```python
from build123d import *

# Parameters (mm, degrees)
BASE_FLANGE1_DEPTH = 2.3
CUT_EXTRUDE2_REACH = 26.82
SKETCH12_W         = 4.6
SKETCH12_H         = 2.3
SKETCH12_W_2       = 3.45
SKETCH6_W          = 3.3
SKETCH6_H          = 7
TAB1_DEPTH         = 2.3
CUT_EXTRUDE1_REACH = 30.373
SKETCH10_R         = 2.5
SKETCH10_R_2       = 1
TAB2_DEPTH         = 2.3


# Sheet-metal steps are written as plain solids
with BuildPart() as part:
    # Sketch1 → Base-Flange1 (new body)
    with BuildSketch(Plane(origin=(0, 0, 0), x_dir=(1, 0, 0), z_dir=(0, 1, 0))):
        with BuildLine():
            Line((-20.6, -10), (20.6, -10))
            ThreePointArc((20.6, -10), (22.014213562, -9.414213562), (22.6, -8))
            Line((22.6, -8), (22.6, 8))
            ThreePointArc((22.6, 8), (22.014213562, 9.414213562), (20.6, 10))
            Line((20.6, 10), (-20.6, 10))
            ThreePointArc((-20.6, 10), (-22.014213562, 9.414213562), (-22.6, 8))
            Line((-22.6, 8), (-22.6, -8))
            ThreePointArc((-22.6, -8), (-22.014213562, -9.414213562), (-20.6, -10))
        make_face()
    extrude(amount=-BASE_FLANGE1_DEPTH)

    # Sketch12 → Cut-Extrude2 (cut, up to next)
    with BuildSketch(Plane(origin=(0, 0, 0), x_dir=(1, 0, 0), z_dir=(0, 1, 0)), mode=Mode.PRIVATE) as cut_extrude2_sk1:
        with Locations((-13, 0)):
            Rectangle(SKETCH12_W, SKETCH12_H)
    cut_extrude2_tool1 = extrude(cut_extrude2_sk1.sketch, amount=-CUT_EXTRUDE2_REACH, mode=Mode.PRIVATE) & part.part
    # Sketch12 → Cut-Extrude2 (cut, up to next)
    with BuildSketch(Plane(origin=(0, 0, 0), x_dir=(1, 0, 0), z_dir=(0, 1, 0)), mode=Mode.PRIVATE) as cut_extrude2_sk2:
        with Locations((7.6, 0)):
            Rectangle(SKETCH12_W, SKETCH12_H)
    cut_extrude2_tool2 = extrude(cut_extrude2_sk2.sketch, amount=-CUT_EXTRUDE2_REACH, mode=Mode.PRIVATE) & part.part
    # Sketch12 → Cut-Extrude2 (cut, up to next)
    with BuildSketch(Plane(origin=(0, 0, 0), x_dir=(1, 0, 0), z_dir=(0, 1, 0)), mode=Mode.PRIVATE) as cut_extrude2_sk3:
        with Locations((-18.3, 3.8)):
            Rectangle(SKETCH12_W, SKETCH12_H)
    cut_extrude2_tool3 = extrude(cut_extrude2_sk3.sketch, amount=-CUT_EXTRUDE2_REACH, mode=Mode.PRIVATE) & part.part
    # Sketch12 → Cut-Extrude2 (cut, up to next)
    with BuildSketch(Plane(origin=(0, 0, 0), x_dir=(1, 0, 0), z_dir=(0, 1, 0)), mode=Mode.PRIVATE) as cut_extrude2_sk4:
        with Locations((18.3, 3.8)):
            Rectangle(SKETCH12_W, SKETCH12_H)
    cut_extrude2_tool4 = extrude(cut_extrude2_sk4.sketch, amount=-CUT_EXTRUDE2_REACH, mode=Mode.PRIVATE) & part.part
    # Sketch12 → Cut-Extrude2 (cut, up to next)
    with BuildSketch(Plane(origin=(0, 0, 0), x_dir=(1, 0, 0), z_dir=(0, 1, 0)), mode=Mode.PRIVATE) as cut_extrude2_sk5:
        with Locations((-18.3, -3.8)):
            Rectangle(SKETCH12_W, SKETCH12_H)
    cut_extrude2_tool5 = extrude(cut_extrude2_sk5.sketch, amount=-CUT_EXTRUDE2_REACH, mode=Mode.PRIVATE) & part.part
    # Sketch12 → Cut-Extrude2 (cut, up to next)
    with BuildSketch(Plane(origin=(0, 0, 0), x_dir=(1, 0, 0), z_dir=(0, 1, 0)), mode=Mode.PRIVATE) as cut_extrude2_sk6:
        with Locations((18.3, -3.8)):
            Rectangle(SKETCH12_W, SKETCH12_H)
    cut_extrude2_tool6 = extrude(cut_extrude2_sk6.sketch, amount=-CUT_EXTRUDE2_REACH, mode=Mode.PRIVATE) & part.part
    # Sketch12 → Cut-Extrude2 (cut, up to next)
    with BuildSketch(Plane(origin=(0, 0, 0), x_dir=(1, 0, 0), z_dir=(0, 1, 0)), mode=Mode.PRIVATE) as cut_extrude2_sk7:
        with Locations((-9.225, 7.6)):
            Rectangle(SKETCH12_W_2, SKETCH12_H)
    cut_extrude2_tool7 = extrude(cut_extrude2_sk7.sketch, amount=-CUT_EXTRUDE2_REACH, mode=Mode.PRIVATE) & part.part
    # Sketch12 → Cut-Extrude2 (cut, up to next)
    with BuildSketch(Plane(origin=(0, 0, 0), x_dir=(1, 0, 0), z_dir=(0, 1, 0)), mode=Mode.PRIVATE) as cut_extrude2_sk8:
        with Locations((-9.225, -7.6)):
            Rectangle(SKETCH12_W_2, SKETCH12_H)
    cut_extrude2_tool8 = extrude(cut_extrude2_sk8.sketch, amount=-CUT_EXTRUDE2_REACH, mode=Mode.PRIVATE) & part.part
    add(cut_extrude2_tool1.solids().sort_by_distance((-13, 0, 0))[0], mode=Mode.SUBTRACT)
    add(cut_extrude2_tool2.solids().sort_by_distance((7.6, 0, 0))[0], mode=Mode.SUBTRACT)
    add(cut_extrude2_tool3.solids().sort_by_distance((-18.3, 0, -3.8))[0], mode=Mode.SUBTRACT)
    add(cut_extrude2_tool4.solids().sort_by_distance((18.3, 0, -3.8))[0], mode=Mode.SUBTRACT)
    add(cut_extrude2_tool5.solids().sort_by_distance((-18.3, 0, 3.8))[0], mode=Mode.SUBTRACT)
    add(cut_extrude2_tool6.solids().sort_by_distance((18.3, 0, 3.8))[0], mode=Mode.SUBTRACT)
    add(cut_extrude2_tool7.solids().sort_by_distance((-9.225, 0, -7.6))[0], mode=Mode.SUBTRACT)
    add(cut_extrude2_tool8.solids().sort_by_distance((-9.225, 0, 7.6))[0], mode=Mode.SUBTRACT)

    # Sketch6 → Tab1 (add)
    with BuildSketch(Plane(origin=(0, 0, 0), x_dir=(1, 0, 0), z_dir=(0, 1, 0))):
        with Locations((-14.5, 13.5)):
            Rectangle(SKETCH6_W, SKETCH6_H)
        with Locations((14.5, 13.5)):
            Rectangle(SKETCH6_W, SKETCH6_H)
        with Locations((14.5, -13.5)):
            Rectangle(SKETCH6_W, SKETCH6_H)
        with Locations((-14.5, -13.5)):
            Rectangle(SKETCH6_W, SKETCH6_H)
    extrude(amount=-TAB1_DEPTH)

    # Sketch9 → Cut-Extrude1 (cut, up to next)
    with BuildSketch(Plane(origin=(0, 0, 0), x_dir=(1, 0, 0), z_dir=(0, 1, 0)), mode=Mode.PRIVATE) as cut_extrude1_sk1:
        Polygon((-12.85, 11.15), (-13.35, 11.15), (-13.35, 13.35), (-13.5, 13.35), (-13.5, 15.85), (-13.35, 15.85), (-13.35, 17), (-12.85, 17), align=None)
    cut_extrude1_tool1 = extrude(cut_extrude1_sk1.sketch, amount=-CUT_EXTRUDE1_REACH, mode=Mode.PRIVATE) & part.part
    # Sketch9 → Cut-Extrude1 (cut, up to next)
    with BuildSketch(Plane(origin=(0, 0, 0), x_dir=(1, 0, 0), z_dir=(0, 1, 0)), mode=Mode.PRIVATE) as cut_extrude1_sk2:
        Polygon((-16.15, 17), (-16.15, 11.15), (-15.65, 11.15), (-15.65, 13.35), (-15.5, 13.35), (-15.5, 15.85), (-15.65, 15.85), (-15.65, 17), align=None)
    cut_extrude1_tool2 = extrude(cut_extrude1_sk2.sketch, amount=-CUT_EXTRUDE1_REACH, mode=Mode.PRIVATE) & part.part
    # Sketch9 → Cut-Extrude1 (cut, up to next)
    with BuildSketch(Plane(origin=(0, 0, 0), x_dir=(1, 0, 0), z_dir=(0, 1, 0)), mode=Mode.PRIVATE) as cut_extrude1_sk3:
        Polygon((-16.15, -11.15), (-15.65, -11.15), (-15.65, -13.35), (-15.5, -13.35), (-15.5, -15.85), (-15.65, -15.85), (-15.65, -17), (-16.15, -17), align=None)
    cut_extrude1_tool3 = extrude(cut_extrude1_sk3.sketch, amount=-CUT_EXTRUDE1_REACH, mode=Mode.PRIVATE) & part.part
    # Sketch9 → Cut-Extrude1 (cut, up to next)
    with BuildSketch(Plane(origin=(0, 0, 0), x_dir=(1, 0, 0), z_dir=(0, 1, 0)), mode=Mode.PRIVATE) as cut_extrude1_sk4:
        Polygon((-12.85, -17), (-12.85, -11.15), (-13.35, -11.15), (-13.35, -13.35), (-13.5, -13.35), (-13.5, -15.85), (-13.35, -15.85), (-13.35, -17), align=None)
    cut_extrude1_tool4 = extrude(cut_extrude1_sk4.sketch, amount=-CUT_EXTRUDE1_REACH, mode=Mode.PRIVATE) & part.part
    # Sketch9 → Cut-Extrude1 (cut, up to next)
    with BuildSketch(Plane(origin=(0, 0, 0), x_dir=(1, 0, 0), z_dir=(0, 1, 0)), mode=Mode.PRIVATE) as cut_extrude1_sk5:
        Polygon((12.85, -11.15), (13.35, -11.15), (13.35, -13.35), (13.5, -13.35), (13.5, -15.85), (13.35, -15.85), (13.35, -17), (12.85, -17), align=None)
    cut_extrude1_tool5 = extrude(cut_extrude1_sk5.sketch, amount=-CUT_EXTRUDE1_REACH, mode=Mode.PRIVATE) & part.part
    # Sketch9 → Cut-Extrude1 (cut, up to next)
    with BuildSketch(Plane(origin=(0, 0, 0), x_dir=(1, 0, 0), z_dir=(0, 1, 0)), mode=Mode.PRIVATE) as cut_extrude1_sk6:
        Polygon((16.15, -17), (16.15, -11.15), (15.65, -11.15), (15.65, -13.35), (15.5, -13.35), (15.5, -15.85), (15.65, -15.85), (15.65, -17), align=None)
    cut_extrude1_tool6 = extrude(cut_extrude1_sk6.sketch, amount=-CUT_EXTRUDE1_REACH, mode=Mode.PRIVATE) & part.part
    # Sketch9 → Cut-Extrude1 (cut, up to next)
    with BuildSketch(Plane(origin=(0, 0, 0), x_dir=(1, 0, 0), z_dir=(0, 1, 0)), mode=Mode.PRIVATE) as cut_extrude1_sk7:
        Polygon((12.85, 17), (12.85, 11.15), (13.35, 11.15), (13.35, 13.35), (13.5, 13.35), (13.5, 15.85), (13.35, 15.85), (13.35, 17), align=None)
    cut_extrude1_tool7 = extrude(cut_extrude1_sk7.sketch, amount=-CUT_EXTRUDE1_REACH, mode=Mode.PRIVATE) & part.part
    # Sketch9 → Cut-Extrude1 (cut, up to next)
    with BuildSketch(Plane(origin=(0, 0, 0), x_dir=(1, 0, 0), z_dir=(0, 1, 0)), mode=Mode.PRIVATE) as cut_extrude1_sk8:
        Polygon((16.15, 11.15), (15.65, 11.15), (15.65, 13.35), (15.5, 13.35), (15.5, 15.85), (15.65, 15.85), (15.65, 17), (16.15, 17), align=None)
    cut_extrude1_tool8 = extrude(cut_extrude1_sk8.sketch, amount=-CUT_EXTRUDE1_REACH, mode=Mode.PRIVATE) & part.part
    add(cut_extrude1_tool1.solids().sort_by_distance((-13.136932, 0, -14.134659))[0], mode=Mode.SUBTRACT)
    add(cut_extrude1_tool2.solids().sort_by_distance((-15.863068, 0, -14.134659))[0], mode=Mode.SUBTRACT)
    add(cut_extrude1_tool3.solids().sort_by_distance((-15.863068, 0, 14.134659))[0], mode=Mode.SUBTRACT)
    add(cut_extrude1_tool4.solids().sort_by_distance((-13.136932, 0, 14.134659))[0], mode=Mode.SUBTRACT)
    add(cut_extrude1_tool5.solids().sort_by_distance((13.136932, 0, 14.134659))[0], mode=Mode.SUBTRACT)
    add(cut_extrude1_tool6.solids().sort_by_distance((15.863068, 0, 14.134659))[0], mode=Mode.SUBTRACT)
    add(cut_extrude1_tool7.solids().sort_by_distance((13.136932, 0, -14.134659))[0], mode=Mode.SUBTRACT)
    add(cut_extrude1_tool8.solids().sort_by_distance((15.863068, 0, -14.134659))[0], mode=Mode.SUBTRACT)

    # Sketch10 → Tab2 (add)
    with BuildSketch(Plane(origin=(0, 0, 0), x_dir=(1, 0, 0), z_dir=(0, 1, 0))):
        with Locations((-23.6, 0)):
            Circle(SKETCH10_R)
        with Locations(Location((-23.6, 0, 0), (0, 0, 270))):
            Circle(SKETCH10_R_2, mode=Mode.SUBTRACT)
    extrude(amount=-TAB2_DEPTH)


solid = part.part
```
Part model, mm, in its own coordinate system. A direction names the side the tool comes from. Give positions to 0.01 mm unless a question says otherwise; leave off trailing zeros. Order: outer loops, then holes, each group sorted by start corner. A loop starts at its lowest first (then second) coordinate and runs counter-clockwise, first axis right, second up. Notation, with made-up numbers: M 50.25,14.25 L 109.25,14.25 A8 ccw 109.25,24.25 Z; hole C 22.25,54.5 d4. An arc over 180 degrees is marked long. Use a Markdown table: item, result. Add a question column.
(1) Mould opens along X. For faces 1 (the face through (12.85, -1, 11)), 2 (the face through (-15.65, -1, 16)), 3 (the face through (-18, -1, 10)) say: +X half, -X half, draft (parallel to the pull), parting line (faces both ways), or undercut.
(2) Saw through at D-D, the plane x = -19. Give the cut face in (y, z).
(3) 3-axis set-ups, long thin cutter, end or side, ignore diameter. For faces 4 (the face through (13.35, -1, -12)), 5 (the face through (16.15, -1, 11)), 6 (the face through (18, -1, -10)), 7 (the face through (8, -1, -1.15)), 8 (the face through (15.5, -1, -15)): which of +Z, -Z, +X, -X, +Y, -Y reach the whole face in a straight line?
(4) Saw through at A-A, the plane x = 8. Give the cut face in (y, z).
(5) Probe line 1 along X through (y, z) = (-1.1, 0); line 2 along X through (y, z) = (-1.55, 3); line 3 along Z through (x, y) = (18.5, -1.8). List the from-to ranges inside material, lowest first. Write a range as [from, to].
(6) Saw through at C-C, the plane z = 0. Give the cut face in (x, y).
(7) Drop flat-ended pins along their axis: P1, Ø0.7, axis at y = -0.5, z = -15, coming from the +X side; P2, Ø0.7, axis at y = -1.5, z = -12, coming from the +X side; P3, Ø0.6, axis at y = -0.5, z = -16.5, coming from the -X side. Give the stop position or say it passes through.
(8) Saw through at B-B, the plane z = -14. Give the cut face in (x, y).
Answer key:
| question | item | result |
|---|---|---|
| 1 | face 1 | undercut |
| 1 | face 2 | -X half |
| 1 | face 3 | draft |
| 2 | outline | M -2.3,-10 L 0,-10 L 0,-4.95 L -2.3,-4.95 Z; M -2.3,-2.65 L 0,-2.65 L 0,2.65 L -2.3,2.65 Z; M -2.3,4.95 L 0,4.95 L 0,10 L -2.3,10 Z |
| 3 | face 4 | -Z, +Y, -Y |
| 3 | face 5 | +Z, +X, +Y, -Y |
| 3 | face 6 | -Z, +X, +Y, -Y |
| 3 | face 7 | +Y, -Y |
| 3 | face 8 | +X, +Y, -Y |
| 4 | outline | M -2.3,-10 L 0,-10 L 0,-1.15 L -2.3,-1.15 Z; M -2.3,1.15 L 0,1.15 L 0,10 L -2.3,10 Z |
| 5 | line 1 | [-26.1, -24.6], [-22.6, -15.3], [-10.7, 5.3], [9.9, 22.6] |
| 5 | line 2 | [-22.6, -20.6], [-16, 16], [20.6, 22.6] |
| 5 | line 3 | [-10, -4.95], [-2.65, 2.65], [4.95, 10] |
| 6 | outline | M -26.1,-2.3 L -24.6,-2.3 L -24.6,0 L -26.1,0 Z; M -22.6,-2.3 L -15.3,-2.3 L -15.3,0 L -22.6,0 Z; M -10.7,-2.3 L 5.3,-2.3 L 5.3,0 L -10.7,0 Z; M 9.9,-2.3 L 22.6,-2.3 L 22.6,0 L 9.9,0 Z |
| 7 | P1 | x = 15.5 |
| 7 | P2 | x = 15.65 |
| 7 | P3 | x = -15.65 |
| 8 | outline | M -15.5,-2.3 L -13.5,-2.3 L -13.5,0 L -15.5,0 Z; M 13.5,-2.3 L 15.5,-2.3 L 15.5,0 L 13.5,0 Z |
